Could you check a few things on this model? Use its own coordinates, in mm. Coordinates: 2 decimals unless noted, no trailing zeros. Loops run counter-clockwise (first coordinate to the right, second up) from the corner with the lowest first, then second, coordinate; pieces in that order, holes last. Notation, with made-up numbers: (1.5, -39) -> (19.5, -39) arc R19 cw to (19.5, -7) -> close; hole circle Ø8 at (35, 54.25). An arc over 180 degrees is marked (long way). One line per question, with ' | ' between items. Start each with the question number.
(1) Suppose I cut it at C-C (x = 7.5). Please give me the cut outline in (y, z).
(2) Suppose I cut it at B-B (z = 19.5). Please give me the cut outline in (x, y).
(3) If I drill on line 1 along X through (y, z) = (9, 28); line 2 along Z through (x, y) = (-35.5, 15); line 3 along Z through (x, y) = (10.5, 35.5), over which ranges is the centre line in solid material (lowest first)?
(4) If we mould it in two halves opening along X, with no side actions, what happens to faces 1 (the face through (1.139, 19.474, -60.627)), 2 (the face through (34.45, 19.47, -22.19)), 3 (the face through (25, 0, 0)), 4 (the face through (28.638, 19.474, 31.143))? For each: pulls with the +X half, pulls with the -X half, needs draft (parallel to the pull), parting line crosses it, or undercut.
(5) I'm going to push flat-ended pins straight in: pin 1 Ø2 at (y, z) = (15, -45) entering from +X; pin 2 Ø0.6 at (x, z) = (40, -17) entering from +Y; pin 3 Ø8 at (y, z) = (27, 40.5) entering from -X. Where does each tip first touch, or does it pass through?
(6) Suppose I cut it at D-D (y = 31.5). Give the number of separate pieces and of enclosed holes in the cut face, plus the area to 3 significant figures.
(7) Suppose I cut it at A-A (x = -21). Please give me the cut outline in (y, z).
```python
from build123d import *

# Parameters (mm, degrees)
SKETCH1_R           = 25.667
SKETCH1_R_2         = 11.666
BOSS_EXTRUDE1_DEPTH = 39.5
SKETCH3_R           = 1
CUT_EXTRUDE2_DEPTH  = 12


with BuildPart() as part:
    # Sketch1 → Boss-Extrude1 (new body)
    with BuildSketch(Plane(origin=(0, 0, 0), x_dir=(0.9998860245595665, 0, -0.015097612078275651), z_dir=(0, 1, 0))):
        with BuildLine():
            Line((-61.169473244, 13.237048576), (-61.945593174, -11.750901277))
            ThreePointArc((-61.945593174, -11.750901277), (-2.965804858, -62.923588573), (59.076056366, -15.509805654))
            Line((59.076056366, -15.509805654), (59.852176295, 9.478144199))
            ThreePointArc((59.852176295, 9.478144199), (0.872387979, 60.650831495), (-61.169473244, 13.237048576))
        make_face()
        with Locations(Location((-1.046708439, -1.136378539, 0), (0, 0, 269.134937682))):
            Circle(SKETCH1_R, mode=Mode.SUBTRACT)
        with Locations(Location((-25.270455744, 29.647637614, 0), (0, 0, 269.134937682))):
            Circle(SKETCH1_R_2, mode=Mode.SUBTRACT)
        with Locations(Location((25.040791951, 28.084981925, 0), (0, 0, 269.134937682))):
            Circle(SKETCH1_R_2, mode=Mode.SUBTRACT)
        with Locations(Location((32.795299128, -20.863621322, 0), (0, 0, 269.134937682))):
            Circle(SKETCH1_R_2, mode=Mode.SUBTRACT)
        with Locations(Location((-36.047749659, -18.725372188, 0), (0, 0, 269.134937682))):
            Circle(SKETCH1_R_2, mode=Mode.SUBTRACT)
    extrude(amount=BOSS_EXTRUDE1_DEPTH)

    # Sketch3 → Cut-Extrude2 (cut)
    with BuildSketch(Plane(origin=(-5.108058327, 40.5, 5.9056653), x_dir=(0.9998727759206764, 0, 0.01595092388174038), z_dir=(0, 1, 0))):
        with Locations(Location((-7.662813984, 48.486882974, 0), (0, 0, 180.913959377))):
            Circle(SKETCH3_R)
        with Locations(Location((15.667378709, 48.486882974, 0), (0, 0, 180.913959377))):
            Circle(SKETCH3_R)
        with Locations(Location((44.967394337, 23.920411988, 0), (0, 0, 180.913959377))):
            Circle(SKETCH3_R)
        with Locations(Location((49.120943166, 2.107633512, 0), (0, 0, 180.913959377))):
            Circle(SKETCH3_R)
        with Locations(Location((30.899804125, -31.507727626, 0), (0, 0, 180.913959377))):
            Circle(SKETCH3_R)
        with Locations(Location((-22.895239399, -31.507727626, 0), (0, 0, 180.913959377))):
            Circle(SKETCH3_R)
        with Locations(Location((-41.116378441, 2.107633512, 0), (0, 0, 180.913959377))):
            Circle(SKETCH3_R)
        with Locations(Location((-36.962829611, 23.920411988, 0), (0, 0, 180.913959377))):
            Circle(SKETCH3_R)
    extrude(amount=-CUT_EXTRUDE2_DEPTH, mode=Mode.SUBTRACT)


solid = part.part
```
Checks:
1) outline: (0, -60.07) -> (39.5, -60.07) -> (39.5, -23.06) -> (0, -23.06) -> close; (0, 25.36) -> (39.5, 25.36) -> (39.5, 62.38) -> (0, 62.38) -> close
2) outline: (-60.06, 0) -> (-47.42, 0) -> (-47.42, 39.5) -> (-60.06, 39.5) -> close; (-24.1, 0) -> (-18.98, 0) -> (-18.98, 39.5) -> (-24.1, 39.5) -> close; (16.92, 0) -> (21.47, 0) -> (21.47, 39.5) -> (16.92, 39.5) -> close; (44.74, 0) -> (58, 0) -> (58, 39.5) -> (44.74, 39.5) -> close
3) line 1: x = -56.71 to -43.5, -28.03 to 24.29, 41.93 to 54.65 | line 2: z = -50.16 to -35.62, -22.91 to 7.6, 30.93 to 52.47 | line 3: z = -59.58 to -42.88, -41.77 to -21.78, 24.08 to 61.88
4) face 1: parting line crosses it | face 2: undercut | face 3: needs draft | face 4: undercut
5) pin 1: stops at x = 41.19 | pin 2: stops at y = 28.5 | pin 3: stops at x = -51.74
6) separate pieces: 1 | enclosed holes: 13 | area: 8,160 mm^2
7) outline: (0, -57.35) -> (39.5, -57.35) -> (39.5, -39.93) -> (0, -39.93) -> close; (0, -18.59) -> (39.5, -18.59) -> (39.5, -14.97) -> (0, -14.97) -> close; (0, 17.28) -> (39.5, 17.28) -> (39.5, 59.65) -> (0, 59.65) -> close
